```python
from build123d import *


with BuildPart() as f1:
    # F0 (on Front) → F1 (revolve)
    with BuildSketch(Plane.XZ):
        with BuildLine():
            Line((16.823175, 27.459773), (19.795203, 27.459773))
            ThreePointArc((19.795203, 27.459773), (14.826528, 32.428447), (9.857854, 27.459773))
            Line((9.857854, 27.459773), (4.83705, 4.592385))
            Line((4.83705, 4.592385), (3.514682, -1.430375))
            Line((3.514682, -1.430375), (6.514682, -1.430375))
            Line((6.514682, -1.430375), (12.833074, 27.346913))
            ThreePointArc((12.833074, 27.346913), (14.770076, 29.455621), (16.823175, 27.459773))
        make_face()
    revolve(axis=Axis((0, 0, 4.655987), (0, 0, 1)))


solid = f1.part
```
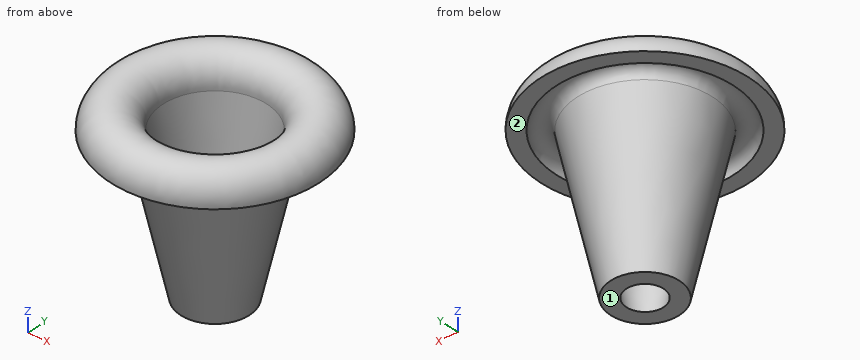
Input: part model. Units: mm. Frame: model coordinates. Face numbers are marked on the shaded views. A direction names the side the tool comes from. Give positions to 0.01 mm unless a question says otherwise; leave off trailing zeros. Order: outer loops, then holes, each group sorted by start corner. A loop starts at its lowest first (then second) coordinate and runs counter-clockwise, first axis right, second up. Notation, with made-up numbers: M 87,-19.5 L 131,-19.5 A25 cw 131,16.5 Z; hole C 51.25,39.25 d2. An arc over 180 degrees is marked long. One line per question, with ' | ' between items.
1) Contact query for flat-ended pins moving along their axis: P1, Ø2, axis at y = -13, z = 27, coming from the +X side; P2, Ø5, axis at y = -4.5, z = 14.5, coming from the -X side; P3, Ø4, axis at x = -6, z = 24, coming from the +Y side. Output: stop coordinate, or through.
Filled in:
P1: stops at x = 15.66 | P2: stops at x = -10.04 | P3: stops at y = 11.56
2) Section A-A on z = 14.5. Output: boundary loops of the cut face in (x, y).
Filled in:
outline: C 0,0 d20.02; hole C 0,0 d14.02
3) Ray query, L1, parallel to Y at x = -7, z = 27.5; L2, parallel to Y at x = -0.5, z = 31; L3, parallel to Y at x = -0.5, z = 30. Return the intervals inside material, ascending.
Filled in:
L1: y = -18.52 to -15.3, -10.75 to -6.94, 6.94 to 10.75, 15.3 to 18.52 | L2: y = -18.31 to -11.33, 11.33 to 18.31 | L3: y = -19.09 to -10.54, 10.54 to 19.09
4) Section C-C on z = 6.5. Output: boundary loops of the cut face in (x, y).
Filled in:
outline: C 0,0 d16.51; hole C 0,0 d10.51
5) Section B-B on z = 28.5. Output: boundary loops of the cut face in (x, y), and give its area (3 significant figures).
Filled in:
outline: C 0,0 d39.37; C 0,0 d26.24; hole C 0,0 d33.06; hole C 0,0 d19.94 | area: 588 mm2
6) Access query for the marked faces 1 and 2. Directions: +Z, -Z, +X, -X, +Y, -Y. A direction counts if a zero-diameter tool reaches every point of the face in a straight line with its end or side. Return the directions, or none.
Filled in:
face 1: -Z, +X, -X, +Y, -Y | face 2: -Z
